Can you work these out from the drawing? Everything is in mm from the part's minimum corner. A direction names the side the tool comes from. Give positions to 0.01 mm unless a question says otherwise; leave off trailing zeros. Write each loop counter-clockwise with the first axis right and the second up, starting at its lowest first coordinate (ties: lowest second). Pieces come first, ordered by that corner, then holes. Notation, with made-up numbers: (-13, -24) - (3, -24) arc R34 cw to (3, 14) - close; hole circle Ø11 at (26.25, -26.5). An arc over 180 degrees is marked (long way). Write each question's results on one line, items separated by ' | '. Start each with the question number.
Item 1: We'd pull the mould along X, two halves only. Please class the marked faces 6, 7, 8 and 9: +X half, -X half, draft (parallel to the pull), parting line (faces both ways), or undercut.
Item 2: Suppose I cut it at A-A on y = 27. List the corners of the cut face in (x, z) for me, then the cut area to 4 significant figures.
Item 3: Suppose I cut it at B-B on x = 10. List the corners of the cut face in (y, z) for me.
Item 4: Please list where these lines run through material, in increasing order: line 1 along X through (y, z) = (9, 2.15); line 2 along Y through (x, z) = (33.75, 1.85); line 3 along Y through (x, z) = (34, 28).
Item 5: Will these pins go through, and if not, where does the flat tip stop? P1, Ø3, axis at y = 6, z = 31.5, coming from the +X side; P2, Ø22, axis at x = 59, z = 10, coming from the +Y side; P3, Ø1, axis at x = 30.5, y = 19.5, coming from the +Z side.
Item 6: Suppose I cut it at C-C on y = 9. List the corners of the cut face in (x, z) for me.
Item 7: Suppose I cut it at D-D on x = 33.75. List the corners of the cut face in (y, z) for me, then the cut area to 3 significant figures.
Item 8: Which directions (+Z, -Z, +X, -X, +Y, -Y) give clear straight access to the entire face, cutting with the end or side of a thin tool? Please do the marked faces 1, 2, 3, 4 and 5.
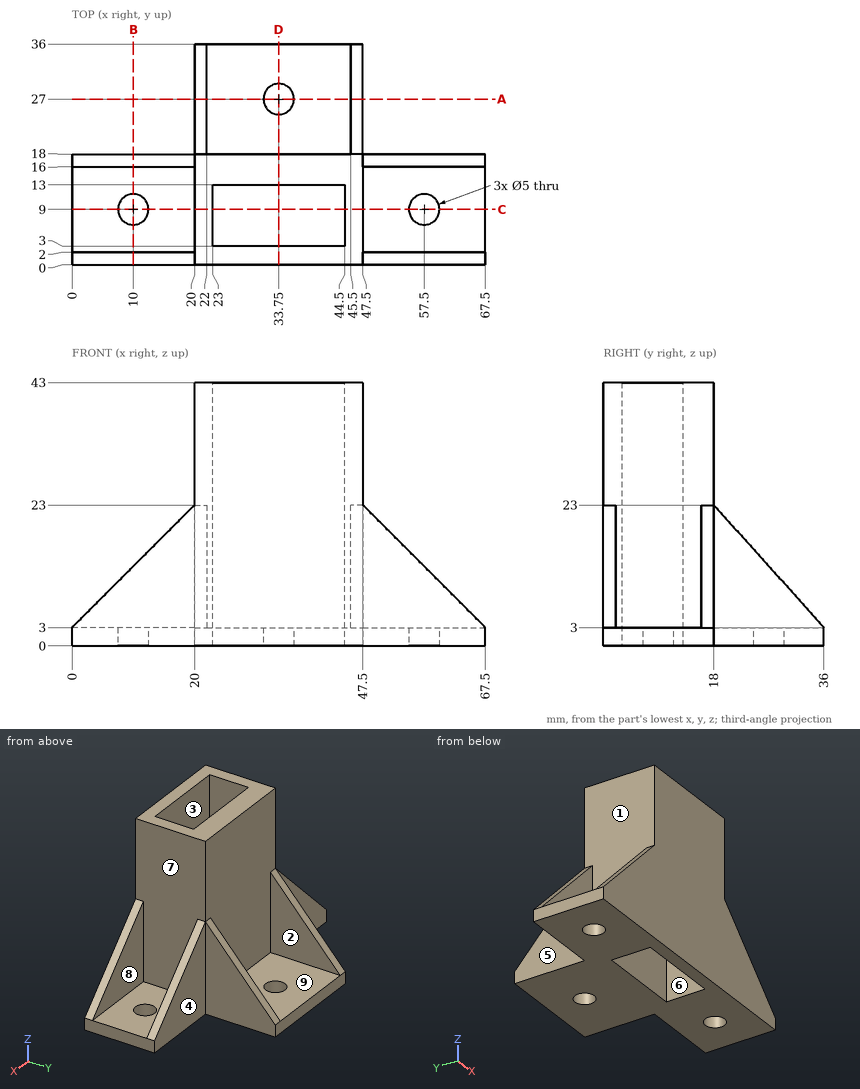
Checked values:
1) face 6: undercut | face 7: +X half | face 8: draft | face 9: undercut
2) outline: (20, 0) - (31.25, 0) - (31.25, 3) - (22, 3) - (22, 13) - (20, 13) - close; (36.25, 0) - (47.5, 0) - (47.5, 13) - (45.5, 13) - (45.5, 3) - (36.25, 3) - close | area: 107.5 mm^2
3) outline: (0, 0) - (6.5, 0) - (6.5, 3) - (2, 3) - (2, 13) - (0, 13) - close; (11.5, 0) - (18, 0) - (18, 13) - (16, 13) - (16, 3) - (11.5, 3) - close
4) line 1: x = 0 to 7.5, 12.5 to 23, 44.5 to 55, 60 to 67.5 | line 2: y = 0 to 3, 13 to 24.5, 29.5 to 36 | line 3: y = 0 to 3, 13 to 18
5) P1: stops at x = 47.5 | P2: stops at y = 18 | P3: stops at z = 3
6) outline: (0, 0) - (7.5, 0) - (7.5, 3) - (0, 3) - close; (12.5, 0) - (23, 0) - (23, 43) - (20, 43) - (20, 3) - (12.5, 3) - close; (44.5, 0) - (55, 0) - (55, 3) - (47.5, 3) - (47.5, 43) - (44.5, 43) - close; (60, 0) - (67.5, 0) - (67.5, 3) - (60, 3) - close
7) outline: (0, 0) - (3, 0) - (3, 43) - (0, 43) - close; (13, 0) - (24.5, 0) - (24.5, 3) - (18, 3) - (18, 43) - (13, 43) - close; (29.5, 0) - (36, 0) - (36, 3) - (29.5, 3) - close | area: 383 mm^2
8) face 1: +Z, -X | face 2: +Z, +Y | face 3: +Z, -Z | face 4: +Z, -Z, +X, +Y | face 5: +Z, -Z, -X, +Y
